Autodesk Inventor part; units mm, degrees
ref_plane "YZ Plane" through (0, 0, 0) normal (1, 0, 0) x (0, 1, 0)
ref_plane "XZ Plane" through (0, 0, 0) normal (0, 1, 0) x (-1, 0, 0)
ref_plane "XY Plane" through (0, 0, 0) normal (0, 0, 1) x (1, 0, 0)
sketch "Boceto1" plane through (0, 0, 0) normal (0, 1, 0) x (-1, 0, 0)
  line L0 (867.2697, 0) -> (-1087.5334, 0) construction
  line L1 (0, 1692.3308) -> (0, -1743.0334) construction
  line L2 (-275, -175) -> (275, -175)
  line L3 (275, -175) -> (275, 175)
  line L4 (275, 175) -> (-275, 175)
  line L5 (-275, 175) -> (-275, -175)
  line L6 (-275, -175) -> (275, 175) construction
  line L7 (275, -175) -> (-275, 175) construction
  point P0 (0, 0)
  dimension "d0" = 550
  dimension "d1" = 350
extrude "Extrusión1" add sketch "Boceto1" along normal blind 25
sketch "Boceto2" plane through (0, 25, 0) normal (0, 1, 0) x (1, 0, 0)
  line L0 (273.5, 173.5) -> (-273.5, 173.5)
  line L1 (-273.5, 173.5) -> (-273.5, -173.5)
  line L2 (-273.5, -173.5) -> (273.5, -173.5)
  line L3 (273.5, -173.5) -> (273.5, 173.5)
  line L4 (273.5, 173.5) -> (-273.5, -173.5) construction
  line L5 (-273.5, 173.5) -> (273.5, -173.5) construction
  line L6 (-275, 175) -> (-275, -175)
  line L7 (-275, -175) -> (275, -175)
  point P0 (0, 0)
  dimension "d4" = 1.5
  dimension "d5" = 1.5
extrude "Extrusión2" cut sketch "Boceto2" against normal blind 23.5
sketch "Boceto3" plane through (273.5, 25, 173.5) normal (0, 0, -1) x (-1, 0, 0)
  line L0 (0, 0) -> (547, 0)
  line L1 (547, 0) -> (0, 0)
  line L2 (0, 0) -> (0, -1.5)
  line L3 (0, -1.5) -> (546.8806, -1.5)
  line L4 (546.8806, -1.5) -> (547, -1.5)
  line L5 (547, -1.5) -> (547, 0)
  point P0 (273.5, -25)
  dimension "d8" = 1.5
extrude "Extrusión3" add sketch "Boceto3" along normal blind 18.5
sketch "Boceto4" plane through (-273.5, 1.5, -173.5) normal (1, 0, 0) x (0, 0, -1)
  line L0 (-328.5, 23.5) -> (0, 23.5)
  line L1 (-328.5, 23.5) -> (-328.5, 22)
  line L2 (0, 23.5) -> (-328.5, 23.5)
  line L3 (-328.5, 23.5) -> (-328.5, 22)
  line L4 (-328.5, 22) -> (0, 22.0229)
  line L5 (0, 23.5) -> (0, 0)
  point P0 (-173.5, -1.5)
  dimension "d11" = 1.5
extrude "Extrusión4" add sketch "Boceto4" along normal blind 18.5
sketch "Boceto5" plane through (-273.5, 1.5, -173.5) normal (0, 0, 1) x (1, 0, 0)
  line L0 (548.5, 23.5) -> (-1.5, 23.5)
  line L1 (546.9606, 23.5) -> (18.5241, 23.5)
  line L2 (18.5, 23.5) -> (18.5, 22.0229)
  line L3 (18.5, 22.0229) -> (547, 22.0229)
  line L4 (547, 23.5) -> (547, 0)
  line L5 (547, 23.5) -> (546.9606, 23.5)
  point P0 (273.5, -1.5)
extrude "Extrusión5" add sketch "Boceto5" along normal blind 18.5
sketch "Boceto6" plane through (273.5, 1.5, -173.5) normal (-1, 0, 0) x (0, 0, 1)
  line L0 (18.5, 23.5) -> (328.5, 23.5)
  line L1 (18.5, 23.5) -> (328.5, 23.5)
  line L2 (328.5, 23.5) -> (328.5, 22.0229)
  line L3 (18.5, 23.5) -> (18.5, 22.0229)
  line L4 (328.5, 22.0229) -> (18.5, 22.0229)
  line L5 (18.5, 22.0229) -> (18.5, 23.5)
  point P0 (173.5, -1.5)
extrude "Extrusión6" add sketch "Boceto6" along normal blind 18.5
sketch "Boceto7" plane through (0, 0, 0) normal (0, -1, 0) x (1, 0, 0)
  line L0 (268.5, -170) -> (-268.5, -170)
  line L1 (-268.5, -170) -> (-268.5, 170)
  line L2 (-268.5, 170) -> (268.5, 170)
  line L3 (268.5, 170) -> (268.5, -170)
  line L4 (268.5, -170) -> (-268.5, 170) construction
  line L5 (-268.5, -170) -> (268.5, 170) construction
  line L6 (-275, 175) -> (275, 175)
  line L7 (-273.5, 173.5) -> (-273.5, -173.5)
  point P0 (0, 0)
  dimension "d18" = 5
  dimension "d19" = 5
extrude "Extrusión7" cut sketch "Boceto7" against normal blind 10
sketch "Boceto8" plane through (0, 25, 0) normal (0, 1, 0) x (1, 0, 0)
  line L0 (-268.5, -170) -> (-268.5, 170)
  line L1 (-268.5, 122.5507) -> (-268.5, 115.1946)
  line L2 (-268.5, -170) -> (268.5, -170)
  line L3 (-149.9016, -170) -> (-169.2021, -170)
  line L4 (-138, -161.5) -> (-135, -161.5)
  line L5 (-138, -168.5) -> (-135, -168.5)
  arc A0 (-138, -161.5) -> (-138, -168.5) centre (-138, -165) ccw
  arc A1 (-135, -168.5) -> (-135, -161.5) centre (-135, -165) ccw
  line L6 (-255, -155) -> (255, -155)
  line L7 (-275, 175) -> (-275, -175)
  line L8 (-288.7354, 0) -> (111.6009, 0) construction
  line L9 (0, -308.0533) -> (0, 294.465) construction
  line L10 (138, -161.5) -> (135, -161.5)
  line L11 (138, -168.5) -> (135, -168.5)
  arc A2 (138, -168.5) -> (138, -161.5) centre (138, -165) ccw
  arc A3 (135, -161.5) -> (135, -168.5) centre (135, -165) ccw
  line L12 (288.7354, 0) -> (-111.6009, 0) construction
  line L13 (-138, 161.5) -> (-135, 161.5)
  line L14 (-138, 168.5) -> (-135, 168.5)
  arc A4 (-138, 168.5) -> (-138, 161.5) centre (-138, 165) ccw
  arc A5 (-135, 161.5) -> (-135, 168.5) centre (-135, 165) ccw
  arc A6 (135, 168.5) -> (135, 161.5) centre (135, 165) ccw
  line L15 (138, 161.5) -> (135, 161.5)
  arc A7 (138, 161.5) -> (138, 168.5) centre (138, 165) ccw
  line L16 (138, 168.5) -> (135, 168.5)
  point P0 (0, 0)
  dimension "d22" = 10
  dimension "d23" = 7
  dimension "d24" = 3
  dimension "d25" = 137
extrude "Extrusión8" cut sketch "Boceto8" against normal blind 10
properties part number "marco"
Input: part model. Units: mm. Frame: model coordinates. A direction names the side the tool comes from. Round coordinates to 2 decimals unless told otherwise and drop trailing zeros. Order: outer loops, then holes, each group sorted by start corner. A loop starts at its lowest first (then second) coordinate and runs counter-clockwise, first axis right, second up.
1. Cut plane B-B, the plane y = 6. Output: boundary loops of the cut face in (x, z).
The answers:
outline: (-275, -175) - (275, -175) - (275, 175) - (-275, 175) - close; hole (-273.5, -173.5) - (273.5, -173.5) - (273.5, 173.5) - (-273.5, 173.5) - close
2. Set-up query: faces 5 (the face through (-275, 12, -2)), 6 (the face through (4, 13, -173.5)). Return all of +Z, -Z, +X, -X, +Y, -Y with unobstructed straight access to the full face (end or side cutting, diameter ignored); none if empty.
The answers:
face 5: +Z, -Z, -X, +Y, -Y
face 6: none
3. Cut plane A-A, the plane x = 111. Output: boundary loops of the cut face in (y, z), then the cut area to 3 significant figures.
The answers:
outline: (0, -175) - (25, -175) - (25, -155) - (23.52, -155) - (23.52, -173.5) - (1.5, -173.5) - (1.5, -170) - (0, -170) - close; (0, 170) - (1.5, 170) - (1.5, 173.5) - (23.5, 173.5) - (23.5, 155) - (25, 155) - (25, 175) - (0, 175) - close
area: 141 mm2
4. Mould query, pull axis X, two halves, no side actions, for faces 1 (the face through (-273.5, 13, -2)), 2 (the face through (1, 25, -156)), 3 (the face through (-4, 13, 173.5)), 4 (the face through (275, 12, 2)). Classes: released by +X, released by -X, zero draft, split by the parting line, or undercut.
The answers:
face 1: undercut
face 2: zero draft
face 3: undercut
face 4: released by +X
5. Cut plane C-C, the plane z = -119. Output: boundary loops of the cut face in (x, y).
The answers:
outline: (-275, 0) - (-268.5, 0) - (-268.5, 1.5) - (-273.5, 1.5) - (-273.5, 23.52) - (-255, 23.52) - (-255, 25) - (-275, 25) - close; (255, 23.52) - (273.5, 23.52) - (273.5, 1.5) - (268.5, 1.5) - (268.5, 0) - (275, 0) - (275, 25) - (255, 25) - close
6. Material intervals for line 1 (Z direction, x = 32.5, y = 15.5); line 2 (X direction, y = 8.75, z = -110.5), sorted ascending.
The answers:
line 1: z = -175 to -173.5, 173.5 to 175
line 2: x = -275 to -273.5, 273.5 to 275
